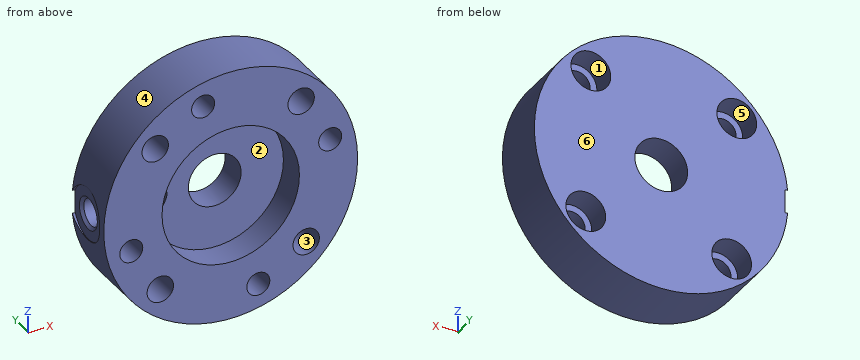
```python
from build123d import *

# Parameters (mm, degrees)
SKETCH1_W         = 19.05
SKETCH1_H         = 8.636
HOLE1_D           = 3.9624
HOLE1_DEPTH       = 8.636
HOLE1_CBORE_D     = 5.969
HOLE1_CBORE_DEPTH = 3.7592
HOLE2_D           = 3.9624
HOLE2_DEPTH       = 8.636
HOLE2_CBORE_D     = 5.969
HOLE2_CBORE_DEPTH = 3.7592
HOLE3_D           = 3.9624
HOLE3_DEPTH       = 8.636
HOLE3_CBORE_D     = 5.969
HOLE3_CBORE_DEPTH = 3.7592
HOLE4_D           = 3.9624
HOLE4_DEPTH       = 8.636
HOLE4_CBORE_D     = 5.969
HOLE4_CBORE_DEPTH = 3.7592
HOLE5_D           = 7.9248
HOLE5_DEPTH       = 8.636
SKETCH13_W        = 10.3124
SKETCH13_H        = 4.318
HOLE6_D           = 3.4544
HOLE6_DEPTH       = 4.318
HOLE7_D           = 3.4544
HOLE7_DEPTH       = 4.318
HOLE8_D           = 3.4544
HOLE8_DEPTH       = 4.318
HOLE9_D           = 3.4544
HOLE9_DEPTH       = 4.318


with BuildPart() as part:
    # Sketch1 → Revolve1 (revolve)
    with BuildSketch(Plane.XY):
        with Locations((9.525, 4.318)):
            Rectangle(SKETCH1_W, SKETCH1_H)
    revolve(axis=Axis((0, 0, 0), (0, 1, 0)))

    # Sketch2 → Cut-Revolve1 (revolve, cut)
    with BuildSketch(Plane.XY):
        Polygon((-19.05, 5.08), (-19.05, 9.04875), (-18.542, 9.04875), (-18.542, 7.493), (-18.11274, 7.06374), (-7.874, 7.06374), (-6.728687177, 5.08), align=None)
    revolve(axis=Axis((-6.728687177, 5.08, 0), (-1, 0, 0)), mode=Mode.SUBTRACT)

    # Hole1
    with Locations(Plane(origin=(0, 8.636, 0), x_dir=(1, 0, 0), z_dir=(0, 1, 0))):
        with Locations((-10.566882591, 11.331594253)):
            CounterBoreHole(HOLE1_D / 2, HOLE1_CBORE_D / 2, HOLE1_CBORE_DEPTH, depth=HOLE1_DEPTH)

    # Hole2
    with Locations(Plane(origin=(0, 8.636, 0), x_dir=(1, 0, 0), z_dir=(0, 1, 0))):
        with Locations((-11.331594253, -10.566882591)):
            CounterBoreHole(HOLE2_D / 2, HOLE2_CBORE_D / 2, HOLE2_CBORE_DEPTH, depth=HOLE2_DEPTH)

    # Hole3
    with Locations(Plane(origin=(0, 8.636, 0), x_dir=(1, 0, 0), z_dir=(0, 1, 0))):
        with Locations((10.566882591, -11.331594253)):
            CounterBoreHole(HOLE3_D / 2, HOLE3_CBORE_D / 2, HOLE3_CBORE_DEPTH, depth=HOLE3_DEPTH)

    # Hole4
    with Locations(Plane(origin=(0, 8.636, 0), x_dir=(1, 0, 0), z_dir=(0, 1, 0))):
        with Locations((11.331594253, 10.566882591)):
            CounterBoreHole(HOLE4_D / 2, HOLE4_CBORE_D / 2, HOLE4_CBORE_DEPTH, depth=HOLE4_DEPTH)

    # Hole5
    with Locations(Plane(origin=(0, 0, 0), x_dir=(-1, 0, 0), z_dir=(0, -1, 0))):
        with Locations((0, 0)):
            Hole(HOLE5_D / 2, depth=HOLE5_DEPTH)

    # Sketch13 → Cut-Revolve2 (revolve, cut)
    with BuildSketch(Plane.XY):
        with Locations((5.1562, 2.159)):
            Rectangle(SKETCH13_W, SKETCH13_H)
    revolve(axis=Axis((0, 0, 0), (0, 1, 0)), mode=Mode.SUBTRACT)

    # Hole6
    with Locations(Plane(origin=(0, 0, 0), x_dir=(-1, 0, 0), z_dir=(0, -1, 0))):
        with Locations((4.140591399, -14.930490242)):
            Hole(HOLE6_D / 2, depth=HOLE6_DEPTH)

    # Hole7
    with Locations(Plane(origin=(0, 0, 0), x_dir=(-1, 0, 0), z_dir=(0, -1, 0))):
        with Locations((-14.930490242, -4.140591399)):
            Hole(HOLE7_D / 2, depth=HOLE7_DEPTH)

    # Hole8
    with Locations(Plane(origin=(0, 0, 0), x_dir=(-1, 0, 0), z_dir=(0, -1, 0))):
        with Locations((-4.140591399, 14.930490242)):
            Hole(HOLE8_D / 2, depth=HOLE8_DEPTH)

    # Hole9
    with Locations(Plane(origin=(0, 0, 0), x_dir=(-1, 0, 0), z_dir=(0, -1, 0))):
        with Locations((14.930490242, 4.140591399)):
            Hole(HOLE9_D / 2, depth=HOLE9_DEPTH)


solid = part.part
```
For this review, take the finished solid that the model builds, in its own axes (mm). Face numbers are marked on the shaded views. A direction names the side the tool comes from. Give positions to 0.01 mm unless a question says otherwise; leave off trailing zeros. Write each loop counter-clockwise with the first axis right and the second up, starting at its lowest first coordinate (ties: lowest second). Pieces come first, ordered by that corner, then holes. Notation, with made-up numbers: M 14,69.5 L 57,69.5 A17 ccw 57,97.5 Z; hole C 29.25,-20 d8. An arc over 180 degrees is marked long. Answer as a JSON object with one key per item and string values. Group by question number.
Item 1: Tool access review of the marked faces 1, 2 and 3: name each direction out of +Z, -Z, +X, -X, +Y, -Y from which nothing blocks a thin tool from reaching the whole face with its end or side.
Item 2: For probe 1 along Z at (x, y) = (-15, 4); probe 2 along Z at (x, y) = (-12, 3); probe 3 along X at (y, z) = (2.75, -12), list the stretches that pass through material, from the lowest coordinate up. Write a range as [from, to].
Item 3: Draft analysis for pull direction X (two halves, no side actions). For the marked faces 4, 5 and 6, state which applies: +X half, -X half, draft (parallel to the pull), parting line (faces both ways), or undercut.
Item 4: Consider section B-B on x = -15.5. Write out the cut boundary in (y, z).
Item 5: For pin 1 Ø2.5 at (y, z) = (5, 2) entering from -X; pin 2 Ø4 at (y, z) = (5.5, -3.5) entering from +X; pin 3 Ø1.7 at (x, z) = (-15.5, -4) entering from -Y, all flat-tipped, find the tip position at first contact; note any pin that passes through.
Item 6: Consider section A-A on x = 0. Write out the cut boundary in (y, z), plus the area to 3 significant figures.
Item 7: Consider section C-C on z = 1. Count the separate pieces of the cut face and the enclosed holes in it, plus the area to 3 significant figures.
Check result:
{
 "1": {"face 1": "+Y", "face 2": "-Y", "face 3": "+Y, -Y"},
 "2": {"probe 1": "z = [-11.74, -5.87], [-2.41, -1.66], [1.66, 11.74]", "probe 2": "z = [-14.8, -12.7], [-9.96, 8.7], [12.43, 14.8]", "probe 3": "x = [-14.8, -12.43], [-8.7, 9.96], [12.7, 14.8]"},
 "3": {"face 4": "parting line", "face 5": "undercut", "face 6": "draft"},
 "4": {"outline": "M 0,-11.07 L 8.64,-11.07 L 8.64,11.07 L 0,11.07 L 0,-2.51 L 4.32,-2.51 L 4.32,-5.77 L 0,-5.77 Z; hole C 5.08,0 d3.97"},
 "5": {"pin 1": "stops at x = -18.54", "pin 2": "stops at x = 18.99", "pin 3": "stops at y = 4.32"},
 "6": {"outline": "M 0,-19.05 L 8.64,-19.05 L 8.64,-3.96 L 4.32,-3.96 L 4.32,-10.31 L 0,-10.31 Z; M 0,10.31 L 4.32,10.31 L 4.32,3.96 L 8.64,3.96 L 8.64,19.05 L 0,19.05 Z", "area": "206 mm^2"},
 "7": {"separate pieces": "3", "enclosed holes": "0", "area": "168 mm^2"}
}
